Input: part model. Units: mm. Frame: model coordinates. Give positions to 0.01 mm unless a question says otherwise; leave off trailing zeros. Loops run counter-clockwise (first coordinate to the right, second up) from the corner with the lowest first, then second, coordinate; pieces in that order, holes last. Notation, with made-up numbers: (64, -3.5) -> (120, -3.5) arc R28 cw to (120, 16.5) -> close; hole circle Ø10 at (-2.75, 33.5). An arc over 180 degrees is marked (long way). Use CSV: the item, a comma, the result in double quotes.
```python
from build123d import *

# Parameters (mm, degrees)
SKETCH1_R           = 12.5
BOSS_EXTRUDE1_DEPTH = 37.500835
SKETCH2_R           = 4.68221709
CUT_EXTRUDE1_DEPTH  = 42.458565167
CHAMFER1_SIZE       = 0.253158
CHAMFER1_SIZE_2     = 0.25155


with BuildPart() as part:
    # Sketch1 → Boss-Extrude1 (new body)
    with BuildSketch(Plane(origin=(0, 0, 0), x_dir=(1, 0, 0), z_dir=(0, 1, 0))):
        with Locations(Location((0, 0, 0), (0, 0, 270))):
            Circle(SKETCH1_R)
    extrude(amount=BOSS_EXTRUDE1_DEPTH)

    # Sketch2 → Cut-Extrude1 (cut, through all)
    with BuildSketch(Plane(origin=(0, 0, 0), x_dir=(1, 0, 0), z_dir=(0, 1, 0))):
        with Locations(Location((0, 0, 0), (0, 0, 270))):
            Circle(SKETCH2_R)
    extrude(amount=CUT_EXTRUDE1_DEPTH, mode=Mode.SUBTRACT)

    # Chamfer1
    # the kernel refuses this chamfer: 0.253158, 0.25155 mm, written as the material it takes off along each edge
    with BuildSketch(Plane(origin=(0, 0, 0), x_dir=(0, 0, 1), z_dir=(-1, 0, 0))) as chamfer1_piece_1:
        Polygon((12.5, CHAMFER1_SIZE), (12.5 - CHAMFER1_SIZE_2, 0), (12.5, 0), align=None)
    revolve(axis=Axis((0, 0, 0), (0, 1, 0)), mode=Mode.SUBTRACT)
    with BuildSketch(Plane(origin=(0, 37.500835, 0), x_dir=(0, 0, 1), z_dir=(-1, 0, 0))) as chamfer1_piece_2:
        Polygon((12.5, -CHAMFER1_SIZE_2), (12.5 - CHAMFER1_SIZE, 0), (12.5, 0), align=None)
    revolve(axis=Axis((0, 37.500835, 0), (0, 1, 0)), mode=Mode.SUBTRACT)
    with BuildSketch(Plane(origin=(0, 0, 0), x_dir=(0, 0, 1), z_dir=(-1, 0, 0))) as chamfer1_piece_3:
        Polygon((4.68221709 + CHAMFER1_SIZE, 0), (4.68221709, CHAMFER1_SIZE_2), (4.68221709, 0), align=None)
    revolve(axis=Axis((0, 0, 0), (0, 1, 0)), mode=Mode.SUBTRACT)
    with BuildSketch(Plane(origin=(0, 37.500835, 0), x_dir=(0, 0, 1), z_dir=(1, 0, 0))) as chamfer1_piece_4:
        Polygon((4.68221709 + CHAMFER1_SIZE_2, 0), (4.68221709, CHAMFER1_SIZE), (4.68221709, 0), align=None)
    revolve(axis=Axis((0, 37.500835, 0), (0, -1, 0)), mode=Mode.SUBTRACT)


solid = part.part
```
1) Section query A-A (x = 0). Return loops of the section in (y, z), then the cut area to 3 significant figures.
From the geometry:
outline,"(0, -12.25) -> (0.25, -12.5) -> (37.25, -12.5) -> (37.5, -12.25) -> (37.5, -4.93) -> (37.25, -4.68) -> (0.25, -4.68) -> (0, -4.94) -> close; (0, 4.94) -> (0.25, 4.68) -> (37.25, 4.68) -> (37.5, 4.93) -> (37.5, 12.25) -> (37.25, 12.5) -> (0.25, 12.5) -> (0, 12.25) -> close"
area,"586 mm^2"
2) Ray query, line 1 (Z direction, x = -0.25, y = 8.5); line 2 (Z direction, x = 4.25, y = 21). Return the intervals inside material, ascending.
From the geometry:
line 1,"z = -12.5 to -4.68, 4.68 to 12.5"
line 2,"z = -11.76 to -1.96, 1.96 to 11.76"
3) Section query B-B (z = 0). Return loops of the section in (x, y), then the cut area to 3 significant figures.
From the geometry:
outline,"(-12.5, 0.25) -> (-12.25, 0) -> (-4.94, 0) -> (-4.68, 0.25) -> (-4.68, 37.25) -> (-4.93, 37.5) -> (-12.25, 37.5) -> (-12.5, 37.25) -> close; (4.68, 0.25) -> (4.94, 0) -> (12.25, 0) -> (12.5, 0.25) -> (12.5, 37.25) -> (12.25, 37.5) -> (4.93, 37.5) -> (4.68, 37.25) -> close"
area,"586 mm^2"
4) Section query C-C (y = 18.5). Return loops of the section in (x, z), then the cut area to 3 significant figures.
From the geometry:
outline,"circle Ø25 at (0, 0); hole circle Ø9.36 at (0, 0)"
area,"422 mm^2"
5) Contact query for flat-ended pins moving along their axis: pin 1 (4 mm diameter, centred on x = 8, y = 5.5, fed in from -Z); pin 2 (1 mm diameter, centred on x = 1.5, y = 33.5, fed in from -Z); pin 3 (3 mm diameter, centred on y = 10.5, z = 9.5, fed in from -X); pin 4 (5.5 mm diameter, centred on x = 0, z = 0, fed in from -Y). Output: stop coordinate, or through.
From the geometry:
pin 1,"stops at z = -10.97"
pin 2,"stops at z = -12.46"
pin 3,"stops at x = -9.6"
pin 4,"passes through"
6) Mould query, pull axis X, two halves, no side actions, for faces 1 (the flat face through (-5.3, 0, -0.2)), 2 (the cylindrical face through (3.755, 18.492, 11.923)), 3 (the cylindrical face through (-4.57, 18.49, -1.02)). Classes: pulls with the +X half, pulls with the -X half, needs draft (parallel to the pull), parting line crosses it, or undercut.
From the geometry:
face 1,"needs draft"
face 2,"parting line crosses it"
face 3,"undercut"
